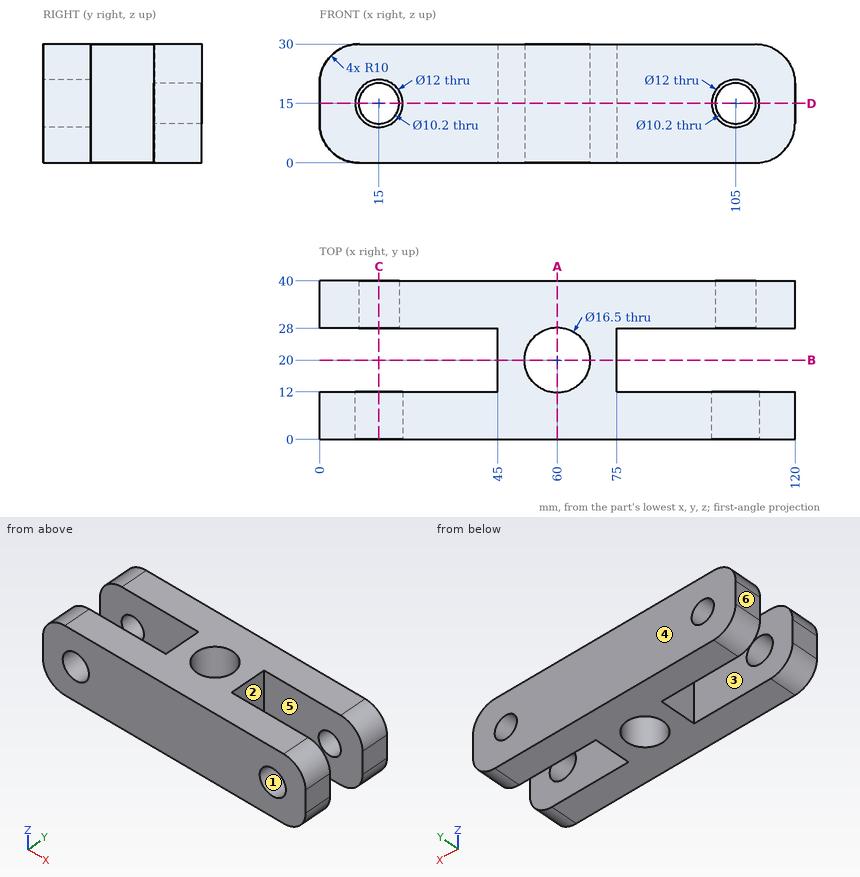
Job drawing, mm, ordinate dimensions from the low corner. One solid piece. A direction names the side the tool comes from. Give positions to 0.01 mm unless a question says otherwise; leave off trailing zeros. Order: outer loops, then holes, each group sorted by start corner. A loop starts at its lowest first (then second) coordinate and runs counter-clockwise, first axis right, second up. Notation, with made-up numbers: (22.5, -14) - (61.5, -14) arc R16 cw to (61.5, 6) - close; hole circle Ø11 at (-23.75, -8.5). An arc over 180 degrees is marked (long way). Answer in a Markdown table with one row per item.
1. Saw through at A-A, the plane x = 60. Give the cut face in (y, z).
Data:
| item | result |
|---|---|
| outline | (0, 0) - (11.75, 0) - (11.75, 30) - (0, 30) - close; (28.25, 0) - (40, 0) - (40, 30) - (28.25, 30) - close |
2. Tool access for the marked faces 1, 2 and 3: list every direction of +Z, -Z, +X, -X, +Y, -Y with a clear straight run to the whole face (end or side of a thin tool).
Data:
| item | result |
|---|---|
| face 1 | -Y |
| face 2 | +Z, -Z, +X |
| face 3 | +Z, -Z, -X |
3. Pull direction Y, two halves, no side cores. Call the marked faces 4, 5 and 6: pulls with the +Y half, pulls with the -Y half, needs draft (parallel to the pull), parting line crosses it, or undercut.
Data:
| item | result |
|---|---|
| face 4 | pulls with the +Y half |
| face 5 | undercut |
| face 6 | needs draft |
4. Saw through at B-B, the plane y = 20. Give the cut face in (x, z), plus the area to 3 significant figures.
Data:
| item | result |
|---|---|
| outline | (45, 0) - (51.75, 0) - (51.75, 30) - (45, 30) - close; (68.25, 0) - (75, 0) - (75, 30) - (68.25, 30) - close |
| area | 405 mm² |
5. Probe probe 1 along Y at (x, z) = (23, 13); probe 2 along Z at (x, y) = (15, 37.25); probe 3 along X at (y, z) = (8.5, 11). List the from-to ranges inside material, lowest first. Write a range as [from, to].
Data:
| item | result |
|---|---|
| probe 1 | y = [0, 12], [28, 40] |
| probe 2 | z = [0, 9.9], [20.1, 30] |
| probe 3 | x = [0, 10.53], [19.47, 100.53], [109.47, 120] |
6. Saw through at D-D, the plane z = 15. Count the separate pieces of the cut face and the enclosed holes in it, plus the area to 3 significant figures.
Data:
| item | result |
|---|---|
| separate pieces | 5 |
| enclosed holes | 1 |
| area | 2,610 mm² |
7. Flat gauge pins, fed straight in: pin 1 (1.5 mm diameter, centred on y = 28, z = 8, fed in from +X); pin 2 (1 mm diameter, centred on y = 13, z = 14, fed in from +X). Where does each tip first touch, or does it go through?
Data:
| item | result |
|---|---|
| pin 1 | stops at x = 119.92 |
| pin 2 | stops at x = 75 |
8. Saw through at C-C, the plane x = 15. Give the cut face in (y, z), plus the area to 3 significant figures.
Data:
| item | result |
|---|---|
| outline | (0, 0) - (12, 0) - (12, 9) - (0, 9) - close; (0, 21) - (12, 21) - (12, 30) - (0, 30) - close; (28, 0) - (40, 0) - (40, 9.9) - (28, 9.9) - close; (28, 20.1) - (40, 20.1) - (40, 30) - (28, 30) - close |
| area | 454 mm² |
